```python
from build123d import *

# Parameters (mm, degrees)
SKETCH1_R           = 1.5
BOSS_EXTRUDE1_DEPTH = 2.6
SKETCH2_W           = 4.15
SKETCH2_H           = 6.3
BOSS_EXTRUDE2_DEPTH = 8.7
SKETCH3_R           = 1.5
BOSS_EXTRUDE3_DEPTH = 1.6
SKETCH4_R           = 1
BOSS_EXTRUDE4_DEPTH = 1.7
SKETCH5_R           = 1.475
CUT_EXTRUDE1_DEPTH  = 2.6
SKETCH6_W           = 4.3
SKETCH6_H           = 5
BOSS_EXTRUDE5_DEPTH = 2
SKETCH7_W           = 7.62
SKETCH7_H           = 2.54
BOSS_EXTRUDE6_DEPTH = 2.54
SKETCH9_W           = 5.7
SKETCH9_H           = 0.6
SKETCH10_W          = 1.95
SKETCH10_H          = 7
CUT_EXTRUDE2_DEPTH  = 2.3


with BuildPart() as part:
    # Sketch1 → Boss-Extrude1 (new body)
    with BuildSketch(Plane(origin=(0, 0, 0), x_dir=(1, 0, 0), z_dir=(0, 1, 0))):
        with BuildLine():
            Line((-9.85, 3.15), (9.85, 3.15))
            ThreePointArc((9.85, 3.15), (13, 0), (9.85, -3.15))
            Line((9.85, -3.15), (-9.85, -3.15))
            ThreePointArc((-9.85, -3.15), (-13, 0), (-9.85, 3.15))
        make_face()
        with Locations((-10.4, 0)):
            Circle(SKETCH1_R, mode=Mode.SUBTRACT)
        with Locations((10.4, 0)):
            Circle(SKETCH1_R, mode=Mode.SUBTRACT)
    extrude(amount=BOSS_EXTRUDE1_DEPTH)

    # Sketch2 → Boss-Extrude2 (add)
    with BuildSketch(Plane(origin=(0, 2.6, 0), x_dir=(1, 0, 0), z_dir=(0, 1, 0))):
        with Locations((-4.975, 0)):
            Rectangle(SKETCH2_W, SKETCH2_H)
        with Locations((4.975, 0)):
            Rectangle(SKETCH2_W, SKETCH2_H)
    extrude(amount=BOSS_EXTRUDE2_DEPTH)

    # Sketch3 → Boss-Extrude3 (add)
    with BuildSketch(Plane.XZ):
        Polygon((-10, 19.85), (-10, 3.15), (-9.85, 3.15), (9.85, 3.15), (10, 3.15), (10, 19.85), align=None)
        with BuildLine():
            ThreePointArc((-9.85, 3.15), (-9.92502128, 3.149106509), (-10, 3.146426545))
            Line((-10, 3.146426545), (-10, 2.175870499))
            Line((-10, 2.175870499), (10, 2.175870499))
            Line((10, 2.175870499), (10, 3.146426545))
            ThreePointArc((10, 3.146426545), (9.92502128, 3.149106509), (9.85, 3.15))
            Line((9.85, 3.15), (-9.85, 3.15))
        make_face()
        with BuildLine():
            ThreePointArc((-10, 3.146426545), (-12.999106509, -0.07502128), (-9.85, -3.15))
            Line((-9.85, -3.15), (9.85, -3.15))
            ThreePointArc((9.85, -3.15), (12.999106509, -0.07502128), (10, 3.146426545))
            Line((10, 3.146426545), (10, 2.175870499))
            Line((10, 2.175870499), (-10, 2.175870499))
            Line((-10, 2.175870499), (-10, 3.146426545))
        make_face()
        with Locations((-10.4, 0)):
            Circle(SKETCH3_R, mode=Mode.SUBTRACT)
        with Locations((10.4, 0)):
            Circle(SKETCH3_R, mode=Mode.SUBTRACT)
    extrude(amount=BOSS_EXTRUDE3_DEPTH)

    # Sketch4 → Boss-Extrude4 (add)
    with BuildSketch(Plane(origin=(0, 0, 0), x_dir=(1, 0, 0), z_dir=(0, 1, 0))):
        with Locations((0, -17.65)):
            Circle(SKETCH4_R)
        with Locations((2.65, -17.65)):
            Circle(SKETCH4_R)
        with Locations((-2.65, -17.65)):
            Circle(SKETCH4_R)
    extrude(amount=BOSS_EXTRUDE4_DEPTH)

    # Sketch5 → Cut-Extrude1 (cut, through all)
    with BuildSketch(Plane(origin=(0, 0, 0), x_dir=(1, 0, 0), z_dir=(0, 1, 0))):
        with Locations((-7.725, -8.575)):
            Circle(SKETCH5_R)
        with Locations((7.725, -8.575)):
            Circle(SKETCH5_R)
    extrude(amount=-CUT_EXTRUDE1_DEPTH, mode=Mode.SUBTRACT)

    # Sketch6 → Boss-Extrude5 (add)
    with BuildSketch(Plane.XZ.offset(1.6)):
        with Locations((0, 6.05)):
            Rectangle(SKETCH6_W, SKETCH6_H)
    extrude(amount=BOSS_EXTRUDE5_DEPTH)

    # Sketch7 → Boss-Extrude6 (add)
    with BuildSketch(Plane.XZ.offset(1.6)):
        with Locations((0, 17.58)):
            Rectangle(SKETCH7_W, SKETCH7_H)
    extrude(amount=BOSS_EXTRUDE6_DEPTH)

    # Sweep1: sweep along a path in Sketch8
    with BuildLine(Plane(origin=(0, 0, 0), x_dir=(0, 0, -1), z_dir=(1, 0, 0))) as sweep1_path:
        Line((-17.58, -4.14), (-17.58, -5.64))
        ThreePointArc((-17.58, -5.64), (-17.433553391, -5.993553391), (-17.08, -6.14))
        Line((-17.08, -6.14), (-10.88, -6.14))
    # Sketch9 → Sweep1 (sweep)
    with BuildSketch(Plane.XZ.offset(4.14)):
        with Locations((0, 17.58)):
            Rectangle(SKETCH9_W, SKETCH9_H)
    sweep(path=sweep1_path.line)

    # Sketch10 → Cut-Extrude2 (cut)
    with BuildSketch(Plane.XZ.offset(6.44)):
        with Locations((-1.275, 14.38)):
            Rectangle(SKETCH10_W, SKETCH10_H)
        with Locations((1.275, 14.38)):
            Rectangle(SKETCH10_W, SKETCH10_H)
    extrude(amount=-CUT_EXTRUDE2_DEPTH, mode=Mode.SUBTRACT)


solid = part.part
```
Input: part model. Units: mm. Frame: model coordinates. A direction names the side the tool comes from. Give positions to 0.01 mm unless a question says otherwise; leave off trailing zeros. Loops run counter-clockwise (first coordinate to the right, second up) from the corner with the lowest first, then second, coordinate; pieces in that order, holes last.
1) Line query: L1, parallel to X at y = 0.9, z = 0; L2, parallel to Y at x = 2.5, z = 16; L3, parallel to Y at x = 8, z = 2.25. Output: solid intervals per line, ascending.
A:
L1: x = -13 to -11.9, -8.9 to 8.9, 11.9 to 13
L2: y = -6.44 to -5.84, -1.6 to 0
L3: y = -1.6 to 2.6
2) Section query B-B on y = -2. Return the cut outline in (x, z), and give its area (3 significant figures).
A:
outline: (-3.81, 16.31) - (3.81, 16.31) - (3.81, 18.85) - (-3.81, 18.85) - close; (-2.15, 3.55) - (2.15, 3.55) - (2.15, 8.55) - (-2.15, 8.55) - close
area: 40.9 mm2
3) Contact query for flat-ended pins moving along their axis: pin 1 (1.3 mm diameter, centred on y = -3, z = 17.5, fed in from +X); pin 2 (1.3 mm diameter, centred on x = -1, z = 6, fed in from -Y); pin 3 (3.5 mm diameter, centred on x = 10.4, z = 0, fed in from +Y); pin 4 (10 mm diameter, centred on x = 1.5, y = 5, fed in from -Z). Output: stop coordinate, or through.
A:
pin 1: stops at x = 3.81
pin 2: stops at y = -3.6
pin 3: stops at y = 2.6
pin 4: stops at z = -3.15
4) Section query C-C on x = 11. Return the cut outline in (y, z).
A:
outline: (-1.6, -2.93) - (2.6, -2.93) - (2.6, -1.37) - (-1.6, -1.37) - close; (-1.6, 1.37) - (2.6, 1.37) - (2.6, 2.93) - (-1.6, 2.93) - close
5) Section query A-A on z = 0. Return the cut outline in (x, y), and give its area (3 significant figures).
A:
outline: (-13, -1.6) - (-11.9, -1.6) - (-11.9, 2.6) - (-13, 2.6) - close; (-8.9, -1.6) - (8.9, -1.6) - (8.9, 2.6) - (7.05, 2.6) - (7.05, 11.3) - (2.9, 11.3) - (2.9, 2.6) - (-2.9, 2.6) - (-2.9, 11.3) - (-7.05, 11.3) - (-7.05, 2.6) - (-8.9, 2.6) - close; (11.9, -1.6) - (13, -1.6) - (13, 2.6) - (11.9, 2.6) - close
area: 156 mm2
6) Mould query, pull axis Z, two halves, no side actions, for faces 4 (the flat face through (0, -3, 3.55)), 5 (the cylindrical face through (0.46, 0.84, 18.54)), 6 (the flat face through (3, 1.7, 18)). Classes: released by +Z, released by -Z, zero draft, split by the parting line, or undercut.
A:
face 4: released by -Z
face 5: undercut
face 6: zero draft
7) Reachability of faces 1 (the flat face through (-10, -1, 12)), 2 (the flat face through (-7.05, 7, 0)), 3 (the flat face through (2.9, 7, 0)) from +Z, -Z, +X, -X, +Y, -Y: full face, straight path, thin tool, end or side. Return the list, or none.
A:
face 1: +Z, -X, +Y, -Y
face 2: +Z, -Z, -X, +Y
face 3: +Z, -Z, +Y
8) Section query D-D on z = 12.5. Return the cut outline in (x, y), and give its area (3 significant figures).
A:
outline: (-10, -1.6) - (10, -1.6) - (10, 0) - (-10, 0) - close; (-2.85, -6.44) - (-2.25, -6.44) - (-2.25, -5.84) - (-2.85, -5.84) - close; (-0.3, -6.44) - (0.3, -6.44) - (0.3, -5.84) - (-0.3, -5.84) - close; (2.25, -6.44) - (2.85, -6.44) - (2.85, -5.84) - (2.25, -5.84) - close
area: 33.1 mm2
